Could you check a few things on this model? Use its own coordinates, in mm. Coordinates: 2 decimals unless noted, no trailing zeros. Loops run counter-clockwise (first coordinate to the right, second up) from the corner with the lowest first, then second, coordinate; pieces in that order, holes last.
from build123d import *

# Parameters (mm, degrees)
SKETCH_1_R          = 57.5
SKETCH_1_R_2        = 44.5
EXTRUDE_1_DEPTH     = 8.6
SKETCH_2_R          = 2.5
CUT_EXTRUDE_1_DEPTH = 82.770777176
CHAMFER_1_SIZE      = 0.5
SKETCH_3_R          = 1.65
CUT_EXTRUDE_2_DEPTH = 82.770777176


with BuildPart() as part:
    # ｽｹｯﾁ1 → ﾎﾞｽ - 押し出し1 (new body)
    with BuildSketch(Plane(origin=(0, 0, 0), x_dir=(1, 0, 0), z_dir=(0, 1, 0))):
        with Locations(Location((0, 0, 0), (0, 0, 90))):
            Circle(SKETCH_1_R)
        with Locations(Location((0, 0, 0), (0, 0, 90))):
            Circle(SKETCH_1_R_2, mode=Mode.SUBTRACT)
    extrude(amount=EXTRUDE_1_DEPTH)

    # ｽｹｯﾁ2 → ｶｯﾄ - 押し出し1 (cut, through all)
    with BuildSketch(Plane(origin=(0, 8.6, 0), x_dir=(1, 0, 0), z_dir=(0, 1, 0))):
        with Locations(Location((-51, 0, 0), (0, 0, 270))):
            Circle(SKETCH_2_R)
        with Locations(Location((0, 51, 0), (0, 0, 270))):
            Circle(SKETCH_2_R)
        with Locations(Location((51, 0, 0), (0, 0, 270))):
            Circle(SKETCH_2_R)
        with Locations(Location((0, -51, 0), (0, 0, 270))):
            Circle(SKETCH_2_R)
    extrude(amount=-CUT_EXTRUDE_1_DEPTH, mode=Mode.SUBTRACT)

    # 面取り1
    chamfer_1_edges = [part.edges().sort_by_distance(p)[0] for p in [
        (0, 0, 57.5),
        (0, 8.6, 57.5),
        (0, 0, 44.5),
        (0, 8.6, 44.5),
    ]]
    chamfer(chamfer_1_edges, length=CHAMFER_1_SIZE)

    # ｽｹｯﾁ3 → ｶｯﾄ - 押し出し2 (cut, through all)
    with BuildSketch(Plane(origin=(0, 8.6, 0), x_dir=(1, 0, 0), z_dir=(0, 1, 0))):
        with Locations(Location((-35, 35, 0), (0, 0, 270))):
            Circle(SKETCH_3_R)
        with Locations(Location((-35, -35, 0), (0, 0, 270))):
            Circle(SKETCH_3_R)
        with Locations(Location((35, -35, 0), (0, 0, 270))):
            Circle(SKETCH_3_R)
        with Locations(Location((35, 35, 0), (0, 0, 270))):
            Circle(SKETCH_3_R)
        with Locations(Location((23.087430662, 44.350541659, 0), (0, 0, 270))):
            Circle(SKETCH_3_R)
        with Locations(Location((44.350541659, -23.087430662, 0), (0, 0, 270))):
            Circle(SKETCH_3_R)
        with Locations(Location((-23.087430662, -44.350541659, 0), (0, 0, 270))):
            Circle(SKETCH_3_R)
        with Locations(Location((-44.350541659, 23.087430662, 0), (0, 0, 270))):
            Circle(SKETCH_3_R)
    extrude(amount=-CUT_EXTRUDE_2_DEPTH, mode=Mode.SUBTRACT)


solid = part.part
(1) I need wall thicknesses on probe 1 along X at (y, z) = (4.5, 0); probe 2 along X at (y, z) = (6, -35); probe 3 along X at (y, z) = (7.25, 24.5). Which ranges of each line are inside material? Lowest first, please.
Answers:
probe 1: x = -57.5 to -53.5, -48.5 to -44.5, 44.5 to 48.5, 53.5 to 57.5
probe 2: x = -45.62 to -36.65, -33.35 to -27.48, 27.48 to 33.35, 36.65 to 45.62
probe 3: x = -52.02 to -37.15, 37.15 to 43.5, 45.2 to 52.02
(2) Imagine slicing it at B-B, the plane z = 0. Write out the boundary of the cut face in (x, y).
Answers:
outline: (-57.5, 0.5) - (-57, 0) - (-53.5, 0) - (-53.5, 8.6) - (-57, 8.6) - (-57.5, 8.1) - close; (-48.5, 0) - (-45, 0) - (-44.5, 0.5) - (-44.5, 8.1) - (-45, 8.6) - (-48.5, 8.6) - close; (44.5, 0.5) - (45, 0) - (48.5, 0) - (48.5, 8.6) - (45, 8.6) - (44.5, 8.1) - close; (53.5, 0) - (57, 0) - (57.5, 0.5) - (57.5, 8.1) - (57, 8.6) - (53.5, 8.6) - close
(3) For pin 1 (2 mm diameter, centred on x = 23.09, z = -44.35, fed in from -Y); pin 2 (5 mm diameter, centred on x = 31.5, y = 1, fed in from +Z); pin 3 (1.5 mm diameter, centred on y = 2, z = 3.5, fed in from +X); pin 4 (1 mm diameter, centred on y = 2.5, z = 26.5, fed in from +X), each with a flat end and sliding along its axis, tell me the tip position at first contact or that it passes through.
Answers:
pin 1: passes through
pin 2: stops at z = 49.65
pin 3: stops at x = 57.43
pin 4: stops at x = 51.29
(4) Imagine slicing it at A-A, the plane x = 0. Write out the boundary of the cut face in (y, z).
Answers:
outline: (0, -57) - (0.5, -57.5) - (8.1, -57.5) - (8.6, -57) - (8.6, -53.5) - (0, -53.5) - close; (0, -48.5) - (8.6, -48.5) - (8.6, -45) - (8.1, -44.5) - (0.5, -44.5) - (0, -45) - close; (0, 45) - (0.5, 44.5) - (8.1, 44.5) - (8.6, 45) - (8.6, 48.5) - (0, 48.5) - close; (0, 53.5) - (8.6, 53.5) - (8.6, 57) - (8.1, 57.5) - (0.5, 57.5) - (0, 57) - close
(5) We'd pull the mould along X, two halves only. Please class faces 1 (the face through (56.133, 4.247, 12.465)), 2 (the face through (38, 8.6, -25)), 3 (the face through (36.115, 4.36, 33.784)): +X half, -X half, draft (parallel to the pull), parting line (faces both ways), or undercut.
Answers:
face 1: parting line
face 2: draft
face 3: undercut
